The figure shows three views and two pictorial views of one solid part (mm, origin at its lowest corner). Answer the questions. A direction names the side the tool comes from. Round coordinates to 2 decimals unless told otherwise and drop trailing zeros. Order: outer loops, then holes, each group sorted by start corner. A loop starts at its lowest first (then second) coordinate and runs counter-clockwise, first axis right, second up. Notation, with made-up numbers: (17, 3.25) -> (24, 3.25) arc R9 ccw to (24, 11.25) -> close; hole circle Ø3 at (65.25, -9). An arc over 180 degrees is marked (long way). Return JSON: item names as keys, results as strings. Group by question number.
(1) The part is cut by section C-C (z = 87). Determine the outline of the cut face in (x, y).
(2) Which of the six approach directions +Z, -Z, +X, -X, +Y, -Y give full straight-line access (tool end or side, diameter ignored) to the marked faces 5, 6 and 7?
(3) Each of these flat-tipped pins is pushed along its axis until it touches: pin 1 (8 mm diameter, centred on x = 7, y = 9.5, fed in from -Z); pin 2 (1.5 mm diameter, centred on x = 28.5, y = 7, fed in from -Z); pin 3 (8 mm diameter, centred on x = 23, y = 20, fed in from +Z); pin 4 (12.5 mm diameter, centred on y = 16.5, z = 22.5, fed in from -X). Where does it stop, or does it pass through?
(4) The part is cut by section B-B (x = 16). Determine the outline of the cut face in (y, z), plus the area to 3 significant figures.
(5) The part is cut by section A-A (y = 13.75). Determine the outline of the cut face in (x, z).
(6) Consider line 1 (X direction, y = 16.75, z = 19.5); line 2 (X direction, y = 9.5, z = 89); line 3 (Z direction, x = 37, y = 11). Determine where each line is inside the solid, lowest interval first. Write a range as [from, to].
(7) Determine the mould class of the marked faces 1, 2, 3 and 4 for opening direction X: +X half, -X half, draft (parallel to the pull), parting line (faces both ways), or undercut.
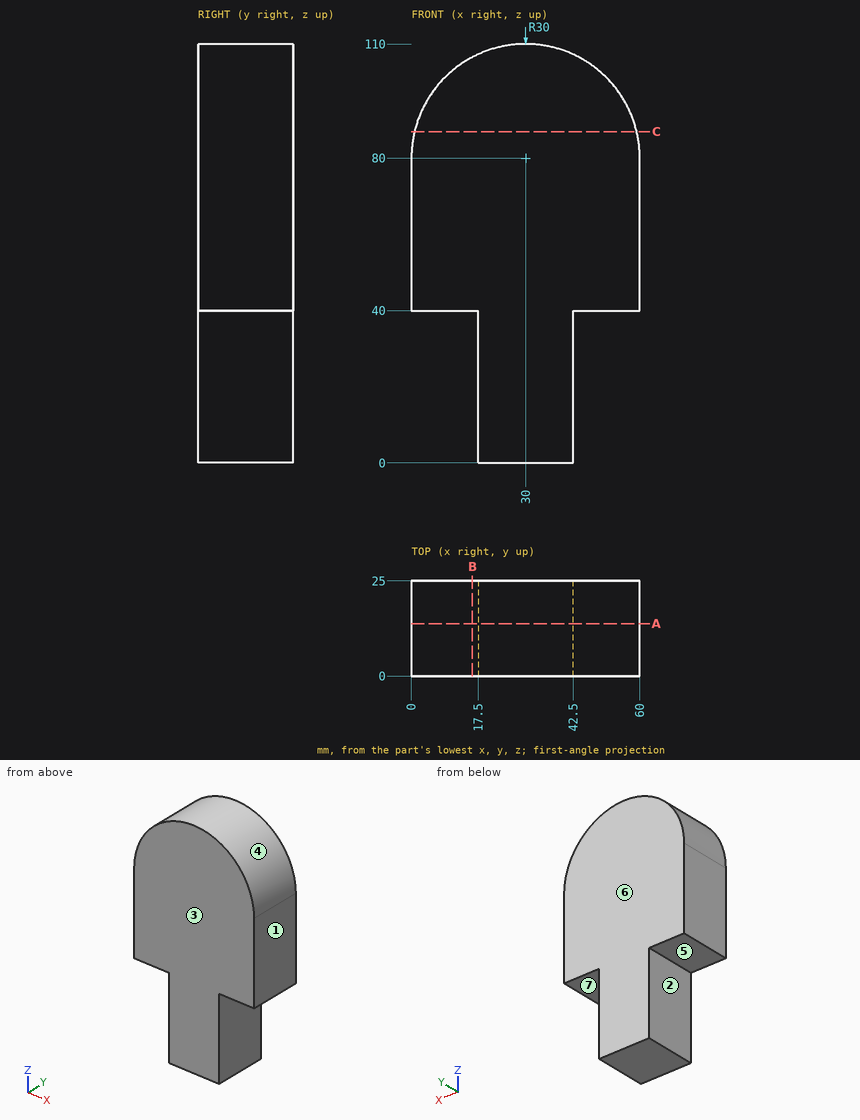
Answer below:
{
 "1": {"outline": "(0.83, 0) -> (59.17, 0) -> (59.17, 25) -> (0.83, 25) -> close"},
 "2": {"face 5": "-Z, -X, +Y, -Y", "face 6": "+Z, -Z, +X, -X, +Y", "face 7": "-Z, +X, +Y, -Y"},
 "3": {"pin 1": "stops at z = 40", "pin 2": "stops at z = 0", "pin 3": "stops at z = 109.85", "pin 4": "stops at x = 17.5"},
 "4": {"outline": "(0, 40) -> (25, 40) -> (25, 106.53) -> (0, 106.53) -> close", "area": "1,660 mm²"},
 "5": {"outline": "(0, 40) -> (17.5, 40) -> (17.5, 0) -> (42.5, 0) -> (42.5, 40) -> (60, 40) -> (60, 80) arc R30 ccw to (0, 80) -> close"},
 "6": {"line 1": "x = [17.5, 42.5]", "line 2": "x = [1.38, 58.62]", "line 3": "z = [0, 109.17]"},
 "7": {"face 1": "+X half", "face 2": "-X half", "face 3": "draft", "face 4": "parting line"}
}
